Geometry check sheet. Reference: drawing and pictorial views, mm from the part's lowest x, y, z. Coordinates: 2 decimals unless noted, no trailing zeros. Loops run counter-clockwise (first coordinate to the right, second up) from the corner with the lowest first, then second, coordinate; pieces in that order, holes last. Notation, with made-up numbers: (40.25, 19) -> (63.25, 19) arc R18 ccw to (63.25, 39) -> close; hole circle Ø11 at (39, 24). An arc over 180 degrees is marked (long way). Answer as a JSON object with one key per item and string values.
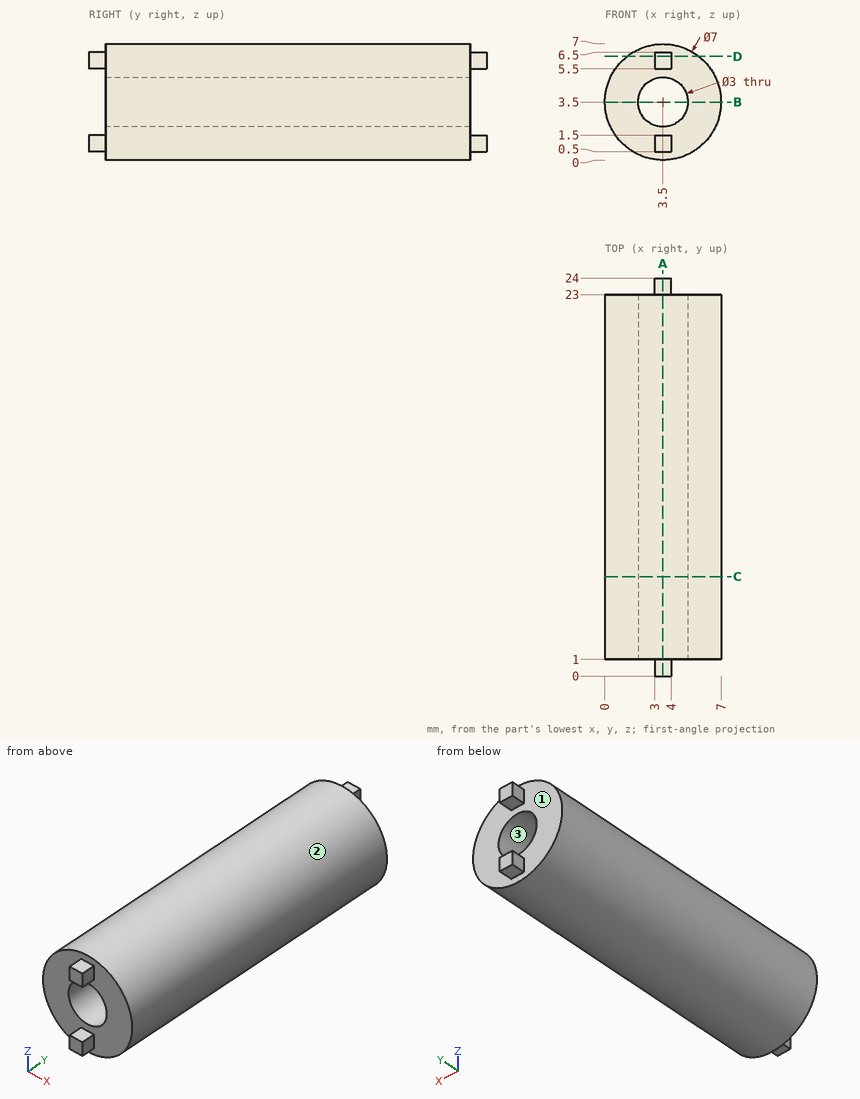
1. Thickness scan on probe 1 along X at (y, z) = (10, 3.5); probe 2 along Y at (x, z) = (2.25, 0.75); probe 3 along Z at (x, y) = (2.5, 12.5). Record the ranges inside material, lowest first. Write a range as from..to.
Evaluation:
{"probe 1": "x = 0..2, 5..7", "probe 2": "y = 1..23", "probe 3": "z = 0.15..2.38, 4.62..6.85"}
2. Mould release check, pull along X, two halves, no side actions. Record for the marked faces 1, 2 and 3: released by +X, released by -X, zero draft, split by the parting line, or undercut.
Evaluation:
{"face 1": "zero draft", "face 2": "split by the parting line", "face 3": "undercut"}
3. Section check A-A, the plane x = 3.5. Record the boundary of the cut face in (y, z), then the cut area to 3 significant figures.
Evaluation:
{"outline": "(0, 0.5) -> (1, 0.5) -> (1, 0) -> (23, 0) -> (23, 0.5) -> (24, 0.5) -> (24, 1.5) -> (23, 1.5) -> (23, 2) -> (1, 2) -> (1, 1.5) -> (0, 1.5) -> close; (0, 5.5) -> (1, 5.5) -> (1, 5) -> (23, 5) -> (23, 5.5) -> (24, 5.5) -> (24, 6.5) -> (23, 6.5) -> (23, 7) -> (1, 7) -> (1, 6.5) -> (0, 6.5) -> close", "area": "92.0 mm^2"}
4. Section check C-C, the plane y = 6. Record the boundary of the cut face in (x, z), then the cut area to 3 significant figures.
Evaluation:
{"outline": "circle Ø7 at (3.5, 3.5); hole circle Ø3 at (3.5, 3.5)", "area": "31.4 mm^2"}
5. Section check D-D, the plane z = 6.25. Record the boundary of the cut face in (x, y).
Evaluation:
{"outline": "(1.33, 1) -> (3, 1) -> (3, 0) -> (4, 0) -> (4, 1) -> (5.67, 1) -> (5.67, 23) -> (4, 23) -> (4, 24) -> (3, 24) -> (3, 23) -> (1.33, 23) -> close"}
6. Section check B-B, the plane z = 3.5. Record the boundary of the cut face in (x, y).
Evaluation:
{"outline": "(0, 1) -> (2, 1) -> (2, 23) -> (0, 23) -> close; (5, 1) -> (7, 1) -> (7, 23) -> (5, 23) -> close"}
7. Depth check by flat-ended pin: P1, Ø0.8, axis at x = 3.5, y = 23.5, coming from the +Z side; P2, Ø0.5, axis at y = 0.5, z = 1, coming from the +X side; P3, Ø0.8, axis at y = 23.5, z = 1, coming from the -X side. Enter the tip coordinate at first touch or a pass-through.
Evaluation:
{"P1": "stops at z = 6.5", "P2": "stops at x = 4", "P3": "stops at x = 3"}
